Input: part model. Units: mm. Frame: model coordinates. Face numbers are marked on the shaded views. Coordinates: 2 decimals unless noted, no trailing zeros. Loops run counter-clockwise (first coordinate to the right, second up) from the corner with the lowest first, then second, coordinate; pieces in that order, holes last. Notation, with made-up numbers: (58, 11.5) -> (90, 11.5) arc R22 ccw to (90, 43.5) -> close; hole circle Ø11 at (-7, 28). An arc over 180 degrees is marked (long way). Answer as a JSON object with one key per item and string values.
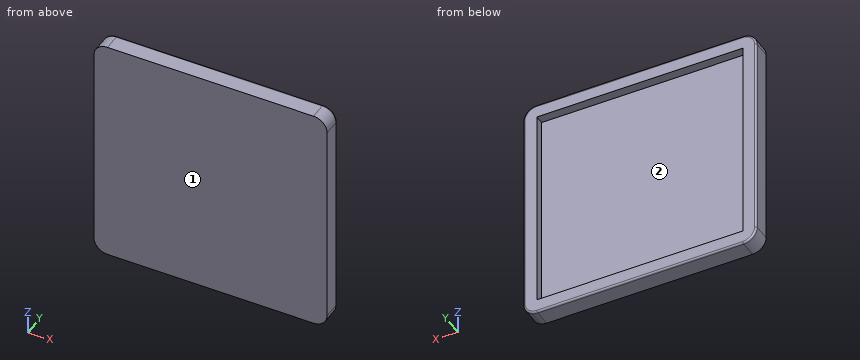
from build123d import *

# Parameters (mm, degrees)
SKETCH1_W           = 128.5
SKETCH1_H           = 128.5
BOSS_EXTRUDE1_DEPTH = 10
SKETCH2_W           = 113.5
SKETCH2_H           = 113.5
CUT_EXTRUDE3_DEPTH  = 5
FILLET1_R           = 7.5
FILLET2_R           = 1


with BuildPart() as part:
    # Sketch1 → Boss-Extrude1 (new body)
    with BuildSketch(Plane(origin=(0, 0, 0), x_dir=(1, 0, 0), z_dir=(0, 1, 0))):
        Rectangle(SKETCH1_W, SKETCH1_H)
    extrude(amount=BOSS_EXTRUDE1_DEPTH)

    # Sketch2 → Cut-Extrude3 (cut)
    with BuildSketch(Plane(origin=(0, 10, 0), x_dir=(1, 0, 0), z_dir=(0, 1, 0))):
        Rectangle(SKETCH2_W, SKETCH2_H)
    extrude(amount=-CUT_EXTRUDE3_DEPTH, mode=Mode.SUBTRACT)

    # Fillet1
    fillet1_edges = [part.edges().sort_by_distance(p)[0] for p in [
        (64.25, 5, 64.25),
        (-64.25, 5, 64.25),
        (-64.25, 5, -64.25),
        (64.25, 5, -64.25),
    ]]
    fillet(fillet1_edges, radius=FILLET1_R)

    # Fillet2
    fillet2_edges = [part.edges().sort_by_distance(p)[0] for p in [
        (64.25, 10, 0),
        (0, 10, 64.25),
        (0, 10, -64.25),
        (-64.25, 10, 0),
        (-62.053300859, 10, 62.053300859),
        (-62.053300859, 10, -62.053300859),
        (62.053300859, 10, -62.053300859),
        (62.053300859, 10, 62.053300859),
    ]]
    fillet(fillet2_edges, radius=FILLET2_R)


solid = part.part
1. Line query: line 1 along X through (y, z) = (6, -50); line 2 along Y through (x, z) = (35, 18). Output: solid intervals per line, ascending.
Reply:
{"line 1": "x = -64.25 to -56.75, 56.75 to 64.25", "line 2": "y = 0 to 5"}
2. Section query B-B (z = -34.5). Return loops of the section in (x, y), plus the area to 3 significant figures.
Reply:
{"outline": "(-64.25, 0) -> (64.25, 0) -> (64.25, 9) arc R1 ccw to (63.25, 10) -> (56.75, 10) -> (56.75, 5) -> (-56.75, 5) -> (-56.75, 10) -> (-63.25, 10) arc R1 ccw to (-64.25, 9) -> close", "area": "717 mm2"}
3. Section query A-A (x = 19.5). Return loops of the section in (y, z), plus the area to 3 significant figures.
Reply:
{"outline": "(0, -64.25) -> (9, -64.25) arc R1 ccw to (10, -63.25) -> (10, -56.75) -> (5, -56.75) -> (5, 56.75) -> (10, 56.75) -> (10, 63.25) arc R1 ccw to (9, 64.25) -> (0, 64.25) -> close", "area": "717 mm2"}
4. Pin query (flat end, axial travel): P1, Ø1, axis at x = 23.5, z = 10.5, coming from the +Y side. Return the tip coordinate at first contact, or that it passes through.
Reply:
{"P1": "stops at y = 5"}
5. Mould query, pull axis Z, two halves, no side actions, for the marked faces 1 and 2. Classes: pulls with the +Z half, pulls with the -Z half, needs draft (parallel to the pull), parting line crosses it, or undercut.
Reply:
{"face 1": "needs draft", "face 2": "undercut"}
